Check sheet for the drawn part. Datum: minimum x, y, z corner. Units: mm. Coordinates: 2 decimals unless noted, no trailing zeros. Loops run counter-clockwise (first coordinate to the right, second up) from the corner with the lowest first, then second, coordinate; pieces in that order, holes last. Notation, with made-up numbers: (-20, 70.5) -> (14, 70.5) arc R31 cw to (14, 106.5) -> close; hole circle Ø9 at (-36.5, 30). An arc over 180 degrees is marked (long way). Use CSV: the item, a comma, the result in double quotes. Start each with the question number.
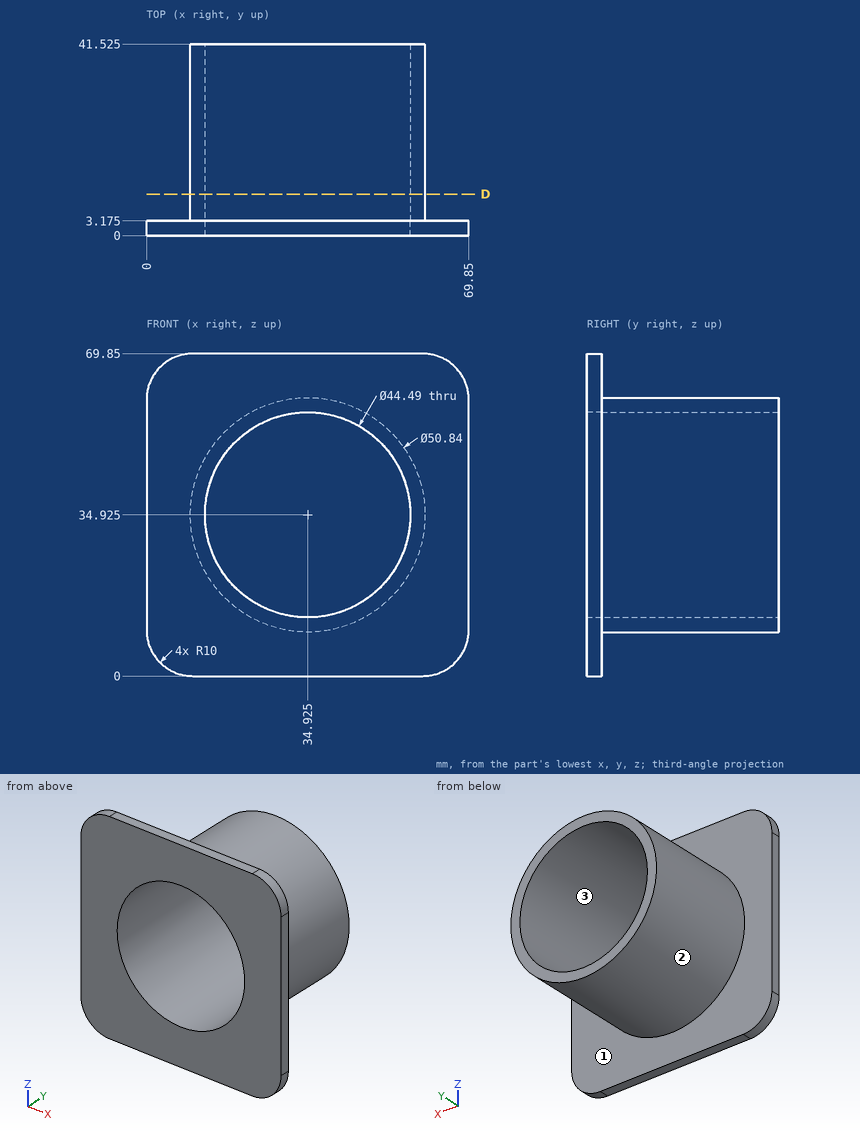
1. Depth check by flat-ended pin: pin 1 (2 mm diameter, centred on x = 23.5, y = 18.5, fed in from +Z); pin 2 (12 mm diameter, centred on y = 13.5, z = 16, fed in from -X); pin 3 (4 mm diameter, centred on x = 19.5, y = 16.5, fed in from +Z). Enter the tip coordinate at first touch or a pass-through.
2. Scan lines: line 1 (Y direction, x = 6, z = 63.5) (3 decimals); line 2 (Z direction, x = 18.5, y = 31) (1 decimal); line 3 (Z direction, x = 34.5, y = 3.5). Record each from-to range of solid material in increasing order.
3. Release check for a two-part mould opening along X. For the marked faces 1, 2 and 3 record: released by +X, released by -X, zero draft, split by the parting line, or undercut.
4. Cross-section at D-D, the plane y = 9. Record the boundary of the cut face in (x, z) (1 decimal).
Solution:
1,pin 1,"stops at z = 58.11"
1,pin 2,"stops at x = 13.04"
1,pin 3,"stops at z = 56.51"
2,line 1,"y = 0 to 3.175"
2,line 2,"z = 15.5 to 19.9, 49.9 to 54.3"
2,line 3,"z = 9.51 to 12.68, 57.17 to 60.34"
3,face 1,"zero draft"
3,face 2,"split by the parting line"
3,face 3,"undercut"
4,outline,"circle Ø50.8 at (34.9, 34.9); hole circle Ø44.5 at (34.9, 34.9)"
